from build123d import *

# Parameters (mm, degrees)
SKIZZE1_W                        = 35
SKIZZE1_H                        = 75
AUFSATZ_LINEAR_AUSTRAGEN1_DEPTH  = 1.5
SKIZZE2_W                        = 11.63
SKIZZE2_H                        = 5
SKIZZE2_W_2                      = 11.62
SKIZZE2_W_3                      = 1.75
SCHNITT_LINEAR_AUSTRAGEN1_DEPTH  = 1.5
SKIZZE13_R                       = 12
SKIZZE13_R_2                     = 11
SCHNITT_LINEAR_AUSTRAGEN10_DEPTH = 20
SKIZZE14_W                       = 27.206049555
SKIZZE14_H                       = 1
AUFSATZ_LINEAR_AUSTRAGEN2_DEPTH  = 1.5
SCHNITT_LINEAR_AUSTRAGEN11_DEPTH = 20


with BuildPart() as part:
    # Skizze1 → Aufsatz-Linear austragen1 (new body)
    with BuildSketch(Plane.XY):
        with Locations((17.5, 37.5)):
            Rectangle(SKIZZE1_W, SKIZZE1_H)
    extrude(amount=AUFSATZ_LINEAR_AUSTRAGEN1_DEPTH)

    # Skizze2 → Schnitt-Linear austragen1 (cut)
    with BuildSketch(Plane.XY.offset(1.5)):
        with Locations((5.815, 2.5)):
            Rectangle(SKIZZE2_W, SKIZZE2_H)
        with Locations((29.19, 2.5)):
            Rectangle(SKIZZE2_W_2, SKIZZE2_H)
        with Locations((17.505, 2.5)):
            Rectangle(SKIZZE2_W_3, SKIZZE2_H)
    extrude(amount=-SCHNITT_LINEAR_AUSTRAGEN1_DEPTH, mode=Mode.SUBTRACT)

    # Skizze13 → Schnitt-Linear austragen10 (cut)
    with BuildSketch(Plane.XY.offset(1.5)):
        with Locations((18, 52.5)):
            Circle(SKIZZE13_R)
        with Locations((18, 52.5)):
            Circle(SKIZZE13_R_2, mode=Mode.SUBTRACT)
    extrude(amount=-SCHNITT_LINEAR_AUSTRAGEN10_DEPTH, mode=Mode.SUBTRACT)


with BuildPart() as schnitt_linear_austragen10_piece_1:
    # of the separate pieces the step leaves, piece 1, a body of its own (schnitt_linear_austragen10_pieces)
    add(part.part.solids().sort_by_distance((11.63, 0, 0))[0])



with BuildPart() as schnitt_linear_austragen10_piece_2:
    # of the separate pieces the step leaves, piece 2, a body of its own (schnitt_linear_austragen10_pieces)
    add(part.part.solids().sort_by_distance((29, 52.5, 0))[0])


with BuildPart() as schnitt_linear_austragen10_piece_1_1:
    add(schnitt_linear_austragen10_piece_1.part)

    add(schnitt_linear_austragen10_piece_2.part)  # Aufsatz-Linear austragen2 merges Schnitt-Linear austragen10 piece 2
    # Skizze14 → Aufsatz-Linear austragen2 (add)
    with BuildSketch(Plane.XY.offset(1.5)):
        with Locations((18.390255325, 52.5)):
            Rectangle(SKIZZE14_W, SKIZZE14_H)
    extrude(amount=-AUFSATZ_LINEAR_AUSTRAGEN2_DEPTH)

    # Skizze15 → Schnitt-Linear austragen11 (cut)
    with BuildSketch(Plane.XY.offset(1.5)):
        Polygon((14.347795458, 17), (13.241164508, 17), (27.231585845, 46.518543423), (29.406174437, 48.771838964), (29.283539592, 48.415672114), (28.532345142, 46.749373442), align=None)
    extrude(amount=-SCHNITT_LINEAR_AUSTRAGEN11_DEPTH, mode=Mode.SUBTRACT)


solid = schnitt_linear_austragen10_piece_1_1.part
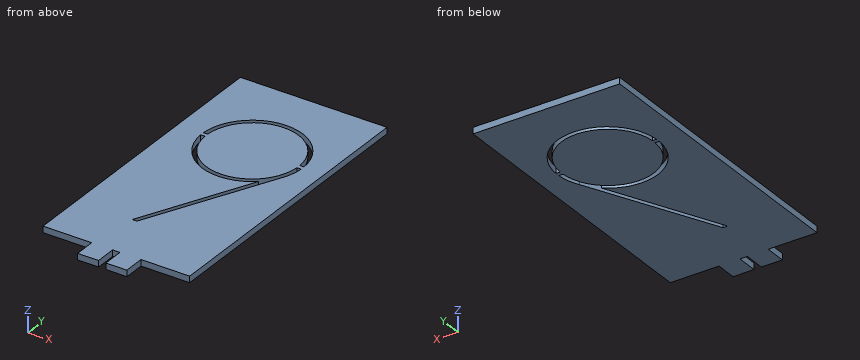
Model file for the job. Use its own axes, mm. Give positions to 0.01 mm unless a question says otherwise; leave off trailing zeros. Loops run counter-clockwise (first coordinate to the right, second up) from the corner with the lowest first, then second, coordinate; pieces in that order, holes last.
1) Saw through at A-A (y = 62). Write the cut outline in (x, z), plus the area to 3 significant figures.
2) Wall check: line 1 (X direction, y = 4.5, z = 0.7); line 2 (X direction, y = 50.5, z = 0.2); line 3 (Y direction, x = 22.5, z = 1). Give the ranges that are in metal, low to high.
3) Saw through at C-C (x = 20). Write the cut outline in (y, z).
4) Saw through at B-B (z = 1.25). Write the cut outline in (x, y), plus the area to 3 significant figures.
5) Flat gauge pins, fed straight in: pin 1 Ø0.5 at (x, z) = (6.5, 0.5) entering from -Y; pin 2 Ø0.8 at (y, z) = (2.5, 1) entering from -X; pin 3 Ø0.8 at (y, z) = (2, 1) entering from +X. Where does each tip first touch, or does it go through?
Answer block:
1. outline: (0, 0) - (10.67, 0) - (10.67, 1.5) - (0, 1.5) - close; (12.45, 0) - (23.55, 0) - (23.55, 1.5) - (12.45, 1.5) - close; (25.33, 0) - (35, 0) - (35, 1.5) - (25.33, 1.5) - close
1. area: 47.1 mm2
2. line 1: x = 11.63 to 16.63, 18.38 to 23.38
2. line 2: x = 0 to 6.17, 7.18 to 28.82, 29.83 to 35
2. line 3: y = 0 to 34.1, 36.54 to 41.38, 42.46 to 62.54, 63.62 to 75
3. outline: (0, 0) - (28.85, 0) - (28.85, 1.5) - (0, 1.5) - close; (31.26, 0) - (40.67, 0) - (40.67, 1.5) - (31.26, 1.5) - close; (41.68, 0) - (63.32, 0) - (63.32, 1.5) - (41.68, 1.5) - close; (64.33, 0) - (75, 0) - (75, 1.5) - (64.33, 1.5) - close
4. outline: (0, 5) - (11.63, 5) - (11.63, 0) - (16.63, 0) - (16.63, 5) - (18.38, 5) - (18.38, 0) - (23.38, 0) - (23.38, 5) - (35, 5) - (35, 75) - (0, 75) - close; hole (6.01, 52) arc R12 ccw to (25.71, 43.3) - (13.24, 17) - (14.35, 17) - (28.53, 46.75) arc R12 ccw to (29.99, 52) - (28.99, 52) arc R11 cw to (7.01, 52) - close; hole (6.01, 53) - (7.01, 53) arc R11 cw to (28.99, 53) - (29.99, 53) arc R12 ccw to start
4. area: 2,400 mm2
5. pin 1: stops at y = 5
5. pin 2: stops at x = 11.63
5. pin 3: stops at x = 23.38
